Read the model definition and answer for the solid it produces. Units are mm, in the model's axes. Round coordinates to 2 decimals unless told otherwise and drop trailing zeros. Write each loop counter-clockwise with the first axis right and the second up, starting at its lowest first coordinate (ties: lowest second). Pieces come first, ordered by that corner, then holes. Notation, with made-up numbers: (24.25, 44) -> (60.25, 44) arc R15 cw to (60.25, 70) -> close; hole circle Ø5 at (23.25, -32.75). An arc over 180 degrees is marked (long way). Return JSON: item names as keys, results as strings. Group by question number.
(1) The mould has two halves that part along X. Classify faces 1 (the flat face through (-1, 1, 10.16)), 2 (the flat face through (-1, 1, 12.7)): released by +X, released by -X, zero draft, split by the parting line, or undercut.
(2) A cutting plane is placed at C-C on z = 1.5. Give the vertices of the cut face in (x, y).
(3) Given pin 1 (2 mm diameter, centred on y = -28, z = 4.5, fed in from +X); pin 2 (1 mm diameter, centred on y = -7, z = 7, fed in from +X); pin 3 (1.5 mm diameter, centred on x = 42.5, z = 2, fed in from +Y), each flat-ended and moving along its own axis, determine where each tip first touches the part or whether it passes through.
(4) Straight lines are drawn through the part: line 1 (Y direction, x = 0, z = 6.75) (3 decimals); line 2 (Z direction, x = 2, y = -33); line 3 (X direction, y = -42, z = 9.25). For each, find the intervals that lie inside material, in ascending order.
```python
from build123d import *

# Parameters (mm, degrees)
F0_R     = 53.975
F1_DEPTH = 12.7
F2_R     = 6.34999
F3_DEPTH = 10.16
F4_R     = 1.27


# Not quite as in the source:
# - a fillet or chamfer is up to 0.001 mm smaller than in the source, because OpenCascade refuses the exact size


with BuildPart() as f1:
    # F0 (on Top) → F1 (new body)
    with BuildSketch(Plane.XY):
        Circle(F0_R)
    extrude(amount=F1_DEPTH)

    # F2 (radius 6.35 in the source; OpenCascade refuses exactly that, so slightly less here)
    f2_edges = [f1.edges().sort_by_distance(p)[0] for p in [
        (53.975, 0, 6.35),
        (-53.975, 0, 0),
        (-53.975, 0, 12.7),
    ]]
    fillet(f2_edges, radius=F2_R)

    # F3 (cut): a face of the model
    f3_faces = [f1.faces().sort_by_distance(p)[0] for p in [
        (0, 0, 0),
    ]]
    extrude(f3_faces, amount=-F3_DEPTH, mode=Mode.SUBTRACT)

    # F4
    f4_edges = [f1.edges().sort_by_distance(p)[0] for p in [
        (-47.62501, 0, 10.16),
    ]]
    fillet(f4_edges, radius=F4_R)


solid = f1.part
```
Checks:
{
 "1": {"face 1": "undercut", "face 2": "zero draft"},
 "2": {"outline": "circle Ø103.45 at (0, 0); hole circle Ø95.25 at (0, 0)"},
 "3": {"pin 1": "stops at x = 46.49", "pin 2": "stops at x = 53.56", "pin 3": "stops at y = 31.87"},
 "4": {"line 1": "y = -53.962 to -47.625, 47.625 to 53.962", "line 2": "z = 10.16 to 12.7", "line 3": "x = -32.77 to -22.34, 22.34 to 32.77"}
}
